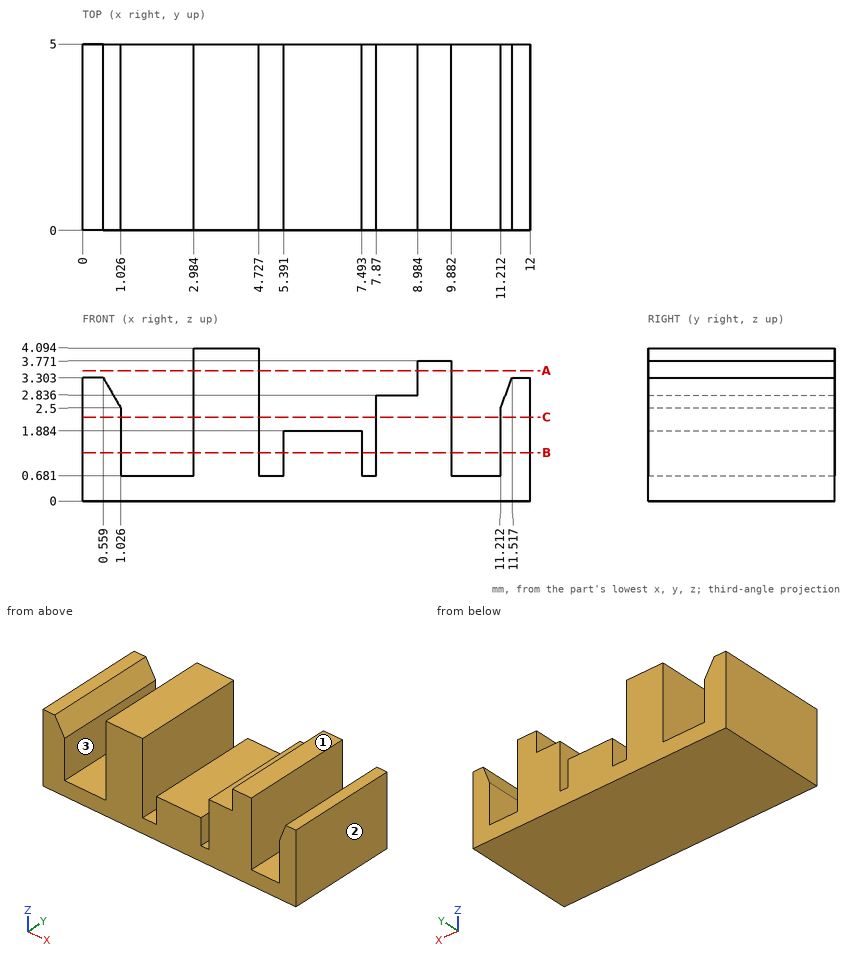
Input: dimensioned drawing with shaded views. Units: mm. Origin: part minimum x, y, z. A direction names the side the tool comes from. Coordinates: 2 decimals unless noted, no trailing zeros. Order: outer loops, then holes, each group sorted by start corner. A loop starts at its lowest first (then second) coordinate and runs counter-clockwise, first axis right, second up.
1. Contact query for flat-ended pins moving along their axis: P1, Ø0.9, axis at x = 8, y = 3, coming from the +Z side; P2, Ø0.6, axis at x = 1.5, y = 2, coming from the +Z side; P3, Ø1.1, axis at x = 6, y = 3, coming from the +Z side. Output: stop coordinate, or through.
Checked values:
P1: stops at z = 2.84
P2: stops at z = 0.68
P3: stops at z = 1.88
2. Cut plane B-B, the plane z = 1.3. Return loops of the section in (x, y) (1 decimal).
Checked values:
outline: (0, 0) - (1, 0) - (1, 5) - (0, 5) - close; (3, 0) - (4.7, 0) - (4.7, 5) - (3, 5) - close; (5.4, 0) - (7.5, 0) - (7.5, 5) - (5.4, 5) - close; (7.9, 0) - (9.9, 0) - (9.9, 5) - (7.9, 5) - close; (11.2, 0) - (12, 0) - (12, 5) - (11.2, 5) - close
3. Cut plane A-A, the plane z = 3.5. Return loops of the section in (x, y) (1 decimal).
Checked values:
outline: (3, 0) - (4.7, 0) - (4.7, 5) - (3, 5) - close; (9, 0) - (9.9, 0) - (9.9, 5) - (9, 5) - close
4. Cut plane C-C, the plane z = 2.25. Return loops of the section in (x, y) (1 decimal).
Checked values:
outline: (0, 0) - (1, 0) - (1, 5) - (0, 5) - close; (3, 0) - (4.7, 0) - (4.7, 5) - (3, 5) - close; (7.9, 0) - (9.9, 0) - (9.9, 5) - (7.9, 5) - close; (11.2, 0) - (12, 0) - (12, 5) - (11.2, 5) - close
5. Access query for the marked faces 1, 2 and 3. Directions: +Z, -Z, +X, -X, +Y, -Y. A direction counts if a zero-diameter tool reaches every point of the face in a straight line with its end or side. Return the directions, or none.
Checked values:
face 1: +Z, +X, +Y, -Y
face 2: +Z, -Z, +X, +Y, -Y
face 3: +Z, +Y, -Y
6. Ray query, line 1 along X through (y, z) = (3.2, 2.35) (1 decimal); line 2 along X through (y, z) = (1.8, 1.3) (1 decimal); line 3 along X through (y, z) = (3, 3.05) (1 decimal). Return the intervals inside material, ascending.
Checked values:
line 1: x = 0 to 1, 3 to 4.7, 7.9 to 9.9, 11.2 to 12
line 2: x = 0 to 1, 3 to 4.7, 5.4 to 7.5, 7.9 to 9.9, 11.2 to 12
line 3: x = 0 to 0.7, 3 to 4.7, 9 to 9.9, 11.4 to 12
